```python
from build123d import *

# Parameters (mm, degrees)
SKETCH8_W               = 97
SKETCH8_H               = 6
SKETCH8_W_2             = 100
BOSS_EXTRUDE1_DEPTH     = 1
CUT_EXTRUDE2_DEPTH      = 223.056299168
CUT_EXTRUDE2_DEPTH_BACK = 223.056299168
SKETCH20_R              = 3
SKETCH20_3_R            = 3
BOSS_EXTRUDE2_DEPTH     = 4


# Read off the part's stored shape, not the designer's step: Cut-Revolve4
with BuildPart() as part:
    # Sketch1 → Revolve2 (revolve)
    with BuildSketch(Plane.XY, mode=Mode.PRIVATE) as revolve2_sk:
        Polygon((-125, 0), (125, 0), (125, 3), (0, 3), (-125, 3), align=None)
    revolve(revolve2_sk.sketch.rotate(Axis((-125, 0, 0), (1, 0, 0)), 180), axis=Axis((-125, 0, 0), (1, 0, 0)))

    # Sketch8 → Boss-Extrude1 (add)
    with BuildSketch(Plane.XY):
        with Locations((-173.5, 0)):
            Rectangle(SKETCH8_W, SKETCH8_H)
        with Locations((172, 0)):
            Rectangle(SKETCH8_W_2, SKETCH8_H)
    extrude(amount=-BOSS_EXTRUDE1_DEPTH)

    # Sketch20 → Cut-Extrude2 (cut, two sides: drawn at the far end of the back side and taken through both)
    with BuildSketch(Plane(origin=(0, 0, -1), x_dir=(-1, 0, 0), z_dir=(0, 0, -1)).offset(-CUT_EXTRUDE2_DEPTH_BACK)):
        with Locations((222, 0)):
            Circle(SKETCH20_R)
        with Locations((-222, 0)):
            Circle(SKETCH20_R)
    extrude(amount=CUT_EXTRUDE2_DEPTH + CUT_EXTRUDE2_DEPTH_BACK, mode=Mode.SUBTRACT)

    # Sketch20<3> → Boss-Extrude2 (add, symmetric)
    with BuildSketch(Plane(origin=(0, 0, -1), x_dir=(-1, 0, 0), z_dir=(0, 0, -1))):
        with Locations((222, 0)):
            Circle(SKETCH20_3_R)
    boss_extrude2 = extrude(amount=BOSS_EXTRUDE2_DEPTH, both=True)

    # Sketch22 → Cut-Revolve3 (revolve, cut)
    with BuildSketch(Plane(origin=(0, 0, -1), x_dir=(-1, 0, 0), z_dir=(0, 0, -1))):
        with BuildLine():
            Line((222, 3), (222, -3))
            ThreePointArc((222, -3), (225, 0), (222, 3))
        make_face()
    revolve(axis=Axis((-222, 3, -1), (0, -1, 0)), mode=Mode.SUBTRACT)


with BuildPart() as cut_revolve3_kept_piece:
    # of the separate pieces the step leaves, the one the design keeps (cut_revolve3_pieces_kept)
    add(part.part.solids().sort_by_distance((-225, 0, 3))[0])

    # Mirror3: Boss-Extrude2 across plane
    add(boss_extrude2.mirror(Plane(origin=(0, 0, 0), x_dir=(0, 0, 1), z_dir=(1, 0, 0))))

    # Cut-Revolve4 outline → Cut-Revolve4 (revolve, cut)
    with BuildSketch(Plane(origin=(222, 0, 0), x_dir=(1, 0, 0), z_dir=(0, -1, 0))):
        with BuildLine():
            Line((0, 2), (0, -5))
            Line((0, -5), (3, -5))
            Line((3, -5), (3, -1.000000003))
            ThreePointArc((3, -1.000000003), (2.121320345, 1.121320342), (0, 2))
        make_face()
    revolve(axis=Axis((222, 0, 0), (0, 0, 1)), mode=Mode.SUBTRACT)


solid = cut_revolve3_kept_piece.part
```
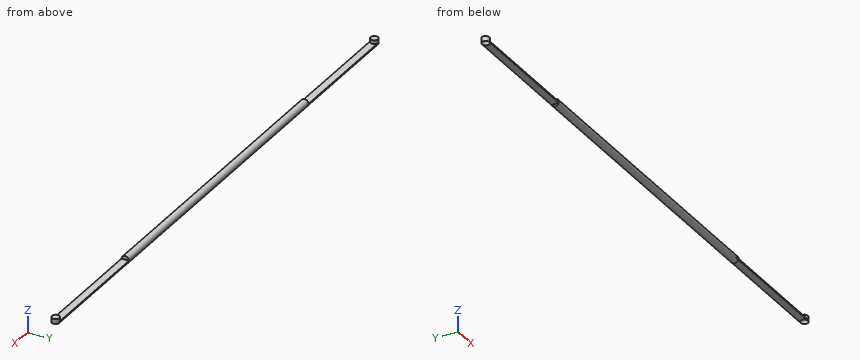
Geometry check sheet. Reference: the model listing, model coordinates, mm. Give positions to 0.01 mm unless a question says otherwise; leave off trailing zeros. Write each loop counter-clockwise with the first axis right and the second up, starting at its lowest first coordinate (ties: lowest second). Pieces come first, ordered by that corner, then holes. Notation, with made-up numbers: (54, 8.25) - (74, 8.25) arc R18 ccw to (74, 18.25) - close; hole circle Ø9 at (43.25, 69.5). An arc over 180 degrees is marked (long way). Use a Markdown table: item, result.
Q1. Section check A-A, the plane y = 0. Enter the section's corners in (x, z).
Computed:
| item | result |
|---|---|
| outline | (-225, -1) arc R3 cw to (-219, -1) - (-125, -1) - (-125, -3) - (125, -3) - (125, -1) - (219, -1) arc R3 cw to (225, -1) - (225, 3) - (219, 3) - (219, 0) - (125, 0) - (125, 3) - (-125, 3) - (-125, 0) - (-219, 0) - (-219, 3) - (-225, 3) - close |
Q2. Go/stop test with flat-tipped pins: P1, Ø1, axis at y = -1, z = -2.5, coming from the +X side; P2, Ø0.9, axis at y = 0.5, z = 1.5, coming from the +X side; P3, Ø2, axis at x = 61, z = 2, coming from the -Y side; P4, Ø3, axis at x = -159.5, y = 1.5, coming from the +Z side. Record where each tip stops, or that it passes through.
Computed:
| item | result |
|---|---|
| P1 | stops at x = 125 |
| P2 | stops at x = 225 |
| P3 | stops at y = -2.83 |
| P4 | stops at z = 0 |
Q3. Section check D-D, the plane x = 55. Enter the section's corners in (y, z).
Computed:
| item | result |
|---|---|
| outline | circle Ø6 at (0, 0) |
Q4. Thickness scan on L1, parallel to X at y = 1.15, z = 0.15; L2, parallel to Z at x = 204, y = 1.95; L3, parallel to Z at x = 107.5, y = -1.1. Record the ranges inside material, lowest first. Write a range as [from, to].
Computed:
| item | result |
|---|---|
| L1 | x = [-224.77, -224.52], [-219.48, -219.23], [-125, 125], [219.23, 219.48], [224.52, 224.77] |
| L2 | z = [-1, 0] |
| L3 | z = [-2.79, 2.79] |
Q5. Section check C-C, the plane z = -2.1. Enter the section's corners in (x, y).
Computed:
| item | result |
|---|---|
| outline | (-125, -2.14) - (125, -2.14) - (125, 2.14) - (-125, 2.14) - close |
Q6. Section check B-B, the plane x = -135. Enter the section's corners in (y, z), then the cut area to 3 significant figures.
Computed:
| item | result |
|---|---|
| outline | (-3, -1) - (3, -1) - (3, 0) - (-3, 0) - close |
| area | 6.00 mm² |
